Geometry: final body of the model. Coordinates: model frame, mm. Give positions to 0.01 mm unless a question says otherwise; leave off trailing zeros. Loops run counter-clockwise (first coordinate to the right, second up) from the corner with the lowest first, then second, coordinate; pieces in that order, holes last. Notation, with made-up numbers: (-25, 7.5) -> (-5, 7.5) arc R27 ccw to (-5, 40.5) -> close; hole circle Ø6 at (44.5, -13.5). An arc over 180 degrees is marked (long way). One line per question, with ' | ' between items. Start each with the question number.
Item 1: Section A-A on x = 2.75. Return loops of the section in (y, z), then the cut area to 3 significant figures.
Item 2: Material intervals for line 1 along Y through (x, z) = (2, 0.75), sorted ascending. Write a range as [from, to].
Item 3: Mould query, pull axis X, two halves, no side actions, for faces 1 (the flat face through (0, -4.2, 4)), 2 (the flat face through (12.5, 0, 0)), 3 (the flat face through (0, -4.5, -6)). Classes: released by +X, released by -X, zero draft, split by the parting line, or undercut.
Item 4: Pin query (flat end, axial travel): P1, Ø2, axis at x = 1, z = 5.5, coming from the -Y side. Return the tip coordinate at first contact, or that it passes through.
from build123d import *

# Parameters (mm, degrees)
SKETCH1_W           = 25
SKETCH1_H           = 25
BOSS_EXTRUDE1_DEPTH = 4.5
SKETCH2_W           = 7
SKETCH2_H           = 16.5
CUT_EXTRUDE1_DEPTH  = 0.3


with BuildPart() as part:
    # Sketch1 → Boss-Extrude1 (new, symmetric)
    with BuildSketch(Plane(origin=(0, 0, 0), x_dir=(1, 0, 0), z_dir=(0, 1, 0))):
        Rectangle(SKETCH1_W, SKETCH1_H)
    extrude(amount=BOSS_EXTRUDE1_DEPTH, both=True)

    # Sketch2 → Cut-Extrude1 (cut)
    with BuildSketch(Plane.XZ.offset(4.5)):
        with Locations((0, 4.25)):
            Rectangle(SKETCH2_W, SKETCH2_H)
    extrude(amount=-CUT_EXTRUDE1_DEPTH, mode=Mode.SUBTRACT)


solid = part.part
Result sheet:
1) outline: (-4.5, -12.5) -> (4.5, -12.5) -> (4.5, 12.5) -> (-4.2, 12.5) -> (-4.2, -4) -> (-4.5, -4) -> close | area: 220 mm²
2) line 1: y = [-4.2, 4.5]
3) face 1: undercut | face 2: released by +X | face 3: zero draft
4) P1: stops at y = -4.2
